Read the model definition and answer for the solid it produces. Units are mm, in the model's axes. A direction names the side the tool comes from. Give positions to 0.01 mm unless a question says otherwise; leave off trailing zeros. Write each loop counter-clockwise with the first axis right and the second up, starting at its lowest first coordinate (ties: lowest second). Pieces come first, ordered by that corner, then holes. Notation, with made-up numbers: M -9,-19 L 49,-19 A24 cw 49,15 Z; hole C 42,78.25 d8. An arc over 180 degrees is marked long. Put each result on its own line as item: value.
from build123d import *

# Parameters (mm, degrees)
F1_DEPTH = 101.6
F2_W     = 50.8
F2_H     = 22.225
F3_DEPTH = 6.35
F4_W     = 25.4
F4_H     = 12.7
F5_DEPTH = 11.43
F7_D     = 6.5278


with BuildPart() as f1:
    # F0 (on Front) → F1 (new body)
    with BuildSketch(Plane.XZ):
        Polygon((25.4, 0), (0, 0), (0, -44.45), (50.8, -44.45), (50.8, -11.43), (25.4, -11.43), align=None)
    extrude(amount=-F1_DEPTH)

    # F2 (on face) → F3 (cut)
    with BuildSketch(Plane(origin=(0, 101.6, 0), x_dir=(-1, 0, 0), z_dir=(0, 1, 0))):
        with Locations((-25.4, -33.3375)):
            Rectangle(F2_W, F2_H)
    extrude(amount=-F3_DEPTH, mode=Mode.SUBTRACT)

    # F4 (on face) → F5 (cut, through all)
    with BuildSketch(Plane.XY):
        with Locations((12.7, 95.25)):
            Rectangle(F4_W, F4_H)
    extrude(amount=-F5_DEPTH, mode=Mode.SUBTRACT)

    # F7 (through all)
    with Locations(Plane.XY):
        with Locations((12.7, 76.2), (12.7, 38.1)):
            Hole(F7_D / 2)


solid = f1.part
(1) Section B-B on y = 76.2 is taken. Determine the outline of the cut face in (x, z).
Result:
outline: M 0,-44.45 L 9.44,-44.45 L 9.44,0 L 0,0 Z; M 15.96,-44.45 L 50.8,-44.45 L 50.8,-11.43 L 25.4,-11.43 L 25.4,0 L 15.96,0 Z
(2) Straight lines are drawn through the part: line 1 along Y through (x, z) = (12.7, -11.5); line 2 along Y through (x, z) = (12.7, -35); line 3 along Y through (x, z) = (6, -10). For each, find the intervals that lie inside material, in ascending order. Write a range as from..to.
Result:
line 1: y = 0..34.84, 41.36..72.94, 79.46..101.6
line 2: y = 0..34.84, 41.36..72.94, 79.46..95.25
line 3: y = 0..88.9
(3) Section C-C on z = -4 is taken. Determine the outline of the cut face in (x, y).
Result:
outline: M 0,0 L 25.4,0 L 25.4,88.9 L 0,88.9 Z; hole C 12.7,38.1 d6.53; hole C 12.7,76.2 d6.53
(4) Given pin 1 Ø3.5 at (x, z) = (14.5, -7) entering from +Y; pin 2 Ø9 at (y, z) = (29, -6) entering from +X, each flat-ended and moving along its own axis, determine where each tip first touches the part or whether it passes through.
Result:
pin 1: stops at y = 88.9
pin 2: stops at x = 25.4
(5) Which of the six approach directions +Z, -Z, +X, -X, +Y, -Y give full straight-line access (tool end or side, diameter ignored) to faces 4 (the face through (26, 98, -22.225)), 5 (the face through (13, 88.9, -6)), 6 (the face through (13, 44, 0))?
Result:
face 4: -Z, +X, -X, +Y
face 5: +Z, +X, -X, +Y
face 6: +Z, +X, -X, +Y, -Y
(6) For a pull along Y with two mould halves and no side action, classify faces 1 (the face through (13.408, 73.014, -22.536)), 2 (the face through (26, 95.25, -33)), 3 (the face through (25.4, 44, -6)) as +Y half, -Y half, draft (parallel to the pull), parting line (faces both ways), or undercut.
Result:
face 1: undercut
face 2: +Y half
face 3: draft
(7) Section D-D on x = 22 is taken. Determine the outline of the cut face in (y, z) (3 decimals), and give its area (3 significant figures).
Result:
outline: M 0,-44.45 L 95.25,-44.45 L 95.25,-22.225 L 101.6,-22.225 L 101.6,-11.43 L 88.9,-11.43 L 88.9,0 L 0,0 Z
area: 4,230 mm²
(8) Section A-A on x = 12.7 is taken. Determine the outline of the cut face in (y, z) (3 decimals), and give its area (3 significant figures).
Result:
outline: M 0,-44.45 L 34.836,-44.45 L 34.836,0 L 0,0 Z; M 41.364,-44.45 L 72.936,-44.45 L 72.936,0 L 41.364,0 Z; M 79.464,-44.45 L 95.25,-44.45 L 95.25,-22.225 L 101.6,-22.225 L 101.6,-11.43 L 88.9,-11.43 L 88.9,0 L 79.464,0 Z
area: 3,650 mm²
